The listing builds one solid part. Answer for the finished solid, in the listing's coordinates (mm). Round coordinates to 2 decimals unless told otherwise and drop trailing zeros. Write each loop counter-clockwise with the first axis right and the second up, starting at its lowest first coordinate (ties: lowest second). Pieces come first, ordered by that corner, then holes. Notation, with made-up numbers: (-24.5, 70) - (28.5, 70) arc R29 ccw to (28.5, 93) - close; hole circle Ø1 at (26, 52.5). An arc over 180 degrees is marked (long way). Answer as CSV lines item,"result". Start each with the question number.
Item 1: A cutting plane is placed at B-B on y = 0.8. State how many separate pieces and enclosed holes the cut face has, and give its area (3 significant figures).
Item 2: Straight lines are drawn through the part: line 1 along X through (y, z) = (0.75, -14.5); line 2 along X through (y, z) = (2.15, 18.5); line 3 along Z through (x, y) = (92.5, 1.1). For each, find the intervals that lie inside material, in ascending order. Write a range as [from, to].
Item 3: Flat-ended cylindrical pins translate along their axes: pin 1 (1 mm diameter, centred on x = -2, y = 2, fed in from +Z); pin 2 (1.5 mm diameter, centred on y = 1, z = -18.5, fed in from -X); pin 3 (0.9 mm diameter, centred on y = 1.5, z = -18.5, fed in from +X). Find the tip coordinate at first contact, or state that the pin passes through.
Item 4: A cutting plane is placed at A-A on x = -46. Determine the outline of the cut face in (y, z).
Item 5: A cutting plane is placed at C-C on x = -67.5. Determine the outline of the cut face in (y, z).
```python
from build123d import *

# Parameters (mm, degrees)
SKETCH1_W           = 200
SKETCH1_H           = 40
BOSS_EXTRUDE1_DEPTH = 3
SKETCH3_W           = 60
SKETCH3_H           = 3
SKETCH3_W_2         = 60.649381746
CUT_EXTRUDE1_DEPTH  = 3
SKETCH4_W           = 13.64
SKETCH4_H           = 8.53
CUT_EXTRUDE2_DEPTH  = 3
SKETCH6_R           = 1.5
CUT_EXTRUDE3_DEPTH  = 3


with BuildPart() as part:
    # Sketch1 → Boss-Extrude1 (new body)
    with BuildSketch(Plane(origin=(0, 0, 0), x_dir=(1, 0, 0), z_dir=(0, 1, 0))):
        Rectangle(SKETCH1_W, SKETCH1_H)
    extrude(amount=BOSS_EXTRUDE1_DEPTH)

    # Sketch3 → Cut-Extrude1 (cut)
    with BuildSketch(Plane(origin=(0, 3, 0), x_dir=(1, 0, 0), z_dir=(0, 1, 0))):
        Polygon((-20, -20), (-20, -17), (-1.5, -17), (-1.5, -15), (-2.75, -15), (-2.75, -12), (-1.5, -12), (-1.5, -10), (1.5, -10), (1.5, -12), (2.75, -12), (2.75, -15), (1.5, -15), (1.5, -17), (20, -17), (20, -20), align=None)
        with Locations((-70, -18.5)):
            Rectangle(SKETCH3_W, SKETCH3_H)
        with Locations((69.675309127, -18.5)):
            Rectangle(SKETCH3_W_2, SKETCH3_H)
        Polygon((85, 17), (100, 17), (100, 20), (60, 20), (60, 17), (82, 17), align=None)
        Polygon((20, 20), (20, 17), (1.5, 17), (1.5, 15), (2.75, 15), (2.75, 12), (1.5, 12), (1.5, 10), (-1.5, 10), (-1.5, 12), (-2.75, 12), (-2.75, 15), (-1.5, 15), (-1.5, 17), (-20, 17), (-20, 20), align=None)
        Polygon((-60, 20), (-60, 17), (-82, 17), (-85, 17), (-100, 17), (-100, 20), align=None)
    extrude(amount=-CUT_EXTRUDE1_DEPTH, mode=Mode.SUBTRACT)

    # Sketch4 → Cut-Extrude2 (cut)
    with BuildSketch(Plane(origin=(0, 3, 0), x_dir=(1, 0, 0), z_dir=(0, 1, 0))):
        with Locations((40.492611387, -10.166269366)):
            Rectangle(SKETCH4_W, SKETCH4_H)
    extrude(amount=-CUT_EXTRUDE2_DEPTH, mode=Mode.SUBTRACT)

    # Sketch6 → Cut-Extrude3 (cut)
    with BuildSketch(Plane.XZ):
        with Locations(Location((92.5, -14.5, 0), (0, 0, 270))):
            Circle(SKETCH6_R)
        with Locations(Location((-77.5, -14.5, 0), (0, 0, 270))):
            Circle(SKETCH6_R)
    extrude(amount=-CUT_EXTRUDE3_DEPTH, mode=Mode.SUBTRACT)


solid = part.part
```
Geometry says:
1,separate pieces,"1"
1,enclosed holes,"3"
1,area,"6,970 mm^2"
2,line 1,"x = [-100, -79], [-76, -2.75], [2.75, 91], [94, 100]"
2,line 2,"x = [-40, -20], [20, 39.35]"
2,line 3,"z = [-17, -16], [-13, 17]"
3,pin 1,"stops at z = 17"
3,pin 2,"stops at x = -60"
3,pin 3,"stops at x = 60"
4,outline,"(0, -20) - (3, -20) - (3, 17) - (0, 17) - close"
5,outline,"(0, -17) - (3, -17) - (3, 17) - (0, 17) - close"
